Work out the finished part from the listing and answer in its coordinate system (mm). Face numbers are marked on the shaded views. A direction names the side the tool comes from. Give positions to 0.01 mm unless a question says otherwise; leave off trailing zeros. Order: outer loops, then holes, each group sorted by start corner. A loop starts at its lowest first (then second) coordinate and runs counter-clockwise, first axis right, second up.
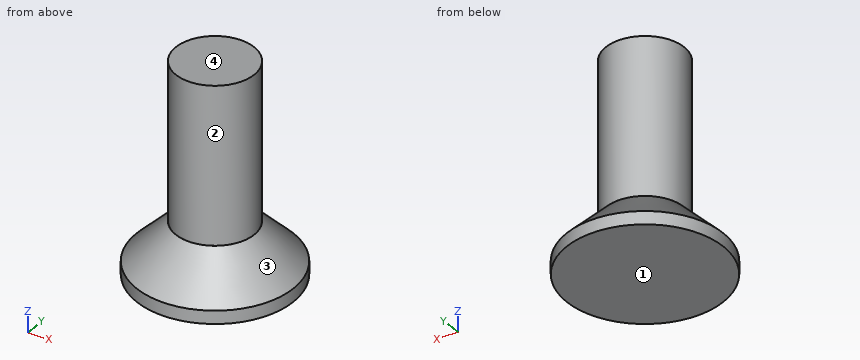
Autodesk Inventor part; units mm, degrees
ref_plane "YZ Plane" through (0, 0, 0) normal (1, 0, 0) x (0, 1, 0)
ref_plane "XZ Plane" through (0, 0, 0) normal (0, 1, 0) x (-1, 0, 0)
ref_plane "XY Plane" through (0, 0, 0) normal (0, 0, 1) x (1, 0, 0)
sketch "スケッチ1" plane through (0, 0, 0) normal (0, 0, 1) x (1, 0, 0)
  circle A0 centre (0, 0) radius 1.5
  dimension "d0" = 3
extrude "押し出し1" add sketch "スケッチ1" along normal blind 8
sketch "スケッチ2" plane through (0, 0, 0) normal (0, 0, -1) x (-1, 0, 0)
  circle A0 centre (0, 0) radius 3
  dimension "d3" = 6
extrude "押し出し2" add sketch "スケッチ2" against normal blind 2
thread "ねじ1"
chamfer "面取り1" distance 1.5 angle 45 1 edges at (3, 0, 2)
properties part number "ネジ皿m3,08" material "鋼、高強度、低合金"
1. Straight lines are drawn through the part: probe 1 along X at (y, z) = (0, 4); probe 2 along X at (y, z) = (0.55, 1.5); probe 3 along Z at (x, y) = (1.65, 0). For each, find the intervals that lie inside material, in ascending order.
Findings below:
probe 1: x = -1.5 to 1.5
probe 2: x = -1.92 to 1.92
probe 3: z = 0 to 1.85
2. The mould has two halves that part along Y. Classify the marked faces 3 and 4: pulls with the +Y half, pulls with the -Y half, needs draft (parallel to the pull), parting line crosses it, or undercut.
Findings below:
face 3: parting line crosses it
face 4: needs draft
3. Which of the six approach directions +Z, -Z, +X, -X, +Y, -Y give full straight-line access (tool end or side, diameter ignored) to the marked faces 1 and 2?
Findings below:
face 1: -Z, +X, -X, +Y, -Y
face 2: +Z
4. Given P1, Ø3, axis at x = -1, z = 7, coming from the -Y side, flat-ended and moving along its own axis, determine where the tip first touches the part or whether it passes through.
Findings below:
P1: stops at y = -1.5
5. The part is cut by section C-C (z = 5.75). Write down the section's boundary in (x, y), then the cut area to 3 significant figures.
Findings below:
outline: circle Ø3 at (0, 0)
area: 7.07 mm2
